from build123d import *

# Parameters (mm, degrees)
PAD_DEPTH       = 5
POCKET_DEPTH    = 5
POCKET001_DEPTH = 2.7
SKETCH001_R     = 6
PAD001_DEPTH    = 10
SKETCH003_R     = 1.75
POCKET002_DEPTH = 15.001
SKETCH_R        = 5.5
POCKET003_DEPTH = 0.28
SKETCH008_R     = 3.108339
PAD002_DEPTH    = 0.28


with BuildPart() as part:
    # Sketch002 → Pad (new body)
    with BuildSketch(Plane(origin=(0, 0, 0), x_dir=(1, 0, 0), z_dir=(0, 0, -1))):
        with BuildLine():
            ThreePointArc((-6.818582, 13.360649), (-8.459114, 12.387227), (-9.962838, 11.213468))
            ThreePointArc((-9.962838, 11.213468), (-11.40037, 11.226378), (-11.365355, 9.789214))
            ThreePointArc((-11.365355, 9.789214), (-12.514173, 8.270155), (-13.461245, 6.617771))
            ThreePointArc((-13.461245, 6.617771), (-14.797088, 6.086557), (-14.221642, 4.769163))
            ThreePointArc((-14.221642, 4.769163), (-14.712665, 2.9219), (-14.964788, 1.027192))
            ThreePointArc((-14.964788, 1.027192), (-15.999972, 0.029665), (-14.968494, -0.971693))
            ThreePointArc((-14.968494, -0.971693), (-14.718057, -2.894616), (-14.221642, -4.769163))
            ThreePointArc((-14.221642, -4.769163), (-14.797088, -6.086557), (-13.461245, -6.617771))
            ThreePointArc((-13.461245, -6.617771), (-12.514173, -8.270155), (-11.365355, -9.789214))
            ThreePointArc((-11.365355, -9.789214), (-11.40037, -11.226378), (-9.962838, -11.213468))
            ThreePointArc((-9.962838, -11.213468), (-8.459114, -12.387227), (-6.818582, -13.360649))
            ThreePointArc((-6.818582, -13.360649), (-6.307429, -14.704296), (-4.981567, -14.148639))
            ThreePointArc((-4.981567, -14.148639), (-3.026004, -14.691606), (-1.015045, -14.965617))
            ThreePointArc((-1.015045, -14.965617), (-0.016678, -15.999991), (0.983842, -14.9677))
            ThreePointArc((0.983842, -14.9677), (3.010688, -14.694753), (4.981567, -14.148639))
            ThreePointArc((4.981567, -14.148639), (6.307429, -14.704296), (6.818582, -13.360649))
            ThreePointArc((6.818582, -13.360649), (8.459114, -12.387227), (9.962838, -11.213468))
            ThreePointArc((9.962838, -11.213468), (11.40037, -11.226378), (11.365355, -9.789214))
            ThreePointArc((11.365355, -9.789214), (12.514173, -8.270155), (13.461245, -6.617771))
            ThreePointArc((13.461245, -6.617771), (14.797088, -6.086557), (14.221642, -4.769163))
            ThreePointArc((14.221642, -4.769163), (14.718057, -2.894616), (14.968494, -0.971693))
            ThreePointArc((14.968494, -0.971693), (15.999972, 0.029665), (14.964788, 1.027192))
            ThreePointArc((14.964788, 1.027192), (14.712665, 2.9219), (14.221642, 4.769163))
            ThreePointArc((14.221642, 4.769163), (14.797088, 6.086557), (13.461245, 6.617771))
            ThreePointArc((13.461245, 6.617771), (12.514173, 8.270155), (11.365355, 9.789214))
            ThreePointArc((11.365355, 9.789214), (11.40037, 11.226378), (9.962838, 11.213468))
            ThreePointArc((9.962838, 11.213468), (8.459114, 12.387227), (6.818582, 13.360649))
            ThreePointArc((6.818582, 13.360649), (6.307429, 14.704296), (4.981567, 14.148639))
            ThreePointArc((4.981567, 14.148639), (3.010688, 14.694753), (0.983842, 14.9677))
            ThreePointArc((0.983842, 14.9677), (-0.016678, 15.999991), (-1.015045, 14.965617))
            ThreePointArc((-1.015045, 14.965617), (-3.026004, 14.691606), (-4.981567, 14.148639))
            ThreePointArc((-4.981567, 14.148639), (-6.307429, 14.704296), (-6.818582, 13.360649))
        make_face()
    extrude(amount=PAD_DEPTH)

    # Sketch006 → Pocket (cut)
    with BuildSketch(Plane.XY):
        with BuildLine():
            ThreePointArc((-9.143797, 7.729592), (-11.061719, 4.581917), (-11.931287, 1))
            Line((-5.91608, 1), (-11.931287, 1))
            ThreePointArc((-4.890405, 3.476196), (-5.543277, 2.296102), (-5.91608, 1))
            Line((-9.143797, 7.729592), (-4.890405, 3.476196))
        make_face()
        with BuildLine():
            ThreePointArc((-11.931287, -1), (-11.061721, -4.581914), (-9.143802, -7.729585))
            Line((-4.890408, -3.476192), (-9.143802, -7.729585))
            ThreePointArc((-5.91608, -1), (-5.543277, -2.2961), (-4.890408, -3.476192))
            Line((-5.91608, -1), (-11.931287, -1))
        make_face()
        with BuildLine():
            ThreePointArc((-1, 11.931287), (-4.581912, 11.061722), (-7.729583, 9.143804))
            Line((-7.729583, 9.143804), (-3.476191, 4.890408))
            ThreePointArc((-1, 5.91608), (-2.296099, 5.543278), (-3.476191, 4.890408))
            Line((-1, 11.931287), (-1, 5.91608))
        make_face()
        with BuildLine():
            ThreePointArc((7.729588, 9.143799), (4.581915, 11.06172), (1, 11.931287))
            Line((1, 11.931287), (1, 5.91608))
            ThreePointArc((3.476194, 4.890406), (2.296101, 5.543277), (1, 5.91608))
            Line((7.729588, 9.143799), (3.476194, 4.890406))
        make_face()
        with BuildLine():
            ThreePointArc((9.143797, -7.729592), (11.061719, -4.581917), (11.931287, -1))
            Line((11.931287, -1), (5.91608, -1))
            ThreePointArc((4.890405, -3.476196), (5.543277, -2.296102), (5.91608, -1))
            Line((4.890405, -3.476196), (9.143797, -7.729592))
        make_face()
        with BuildLine():
            ThreePointArc((1, -11.931287), (4.581912, -11.061722), (7.729583, -9.143804))
            Line((3.476191, -4.890408), (7.729583, -9.143804))
            ThreePointArc((1, -5.91608), (2.296099, -5.543278), (3.476191, -4.890408))
            Line((1, -5.91608), (1, -11.931287))
        make_face()
        with BuildLine():
            ThreePointArc((-7.729589, -9.143799), (-4.581916, -11.06172), (-1, -11.931287))
            Line((-1, -5.91608), (-1, -11.931287))
            ThreePointArc((-3.476194, -4.890406), (-2.296101, -5.543277), (-1, -5.91608))
            Line((-3.476194, -4.890406), (-7.729589, -9.143799))
        make_face()
        with BuildLine():
            ThreePointArc((11.931287, 1), (11.061721, 4.581914), (9.143802, 7.729586))
            Line((9.143802, 7.729586), (4.890407, 3.476193))
            ThreePointArc((5.91608, 1), (5.543277, 2.2961), (4.890407, 3.476193))
            Line((11.931287, 1), (5.91608, 1))
        make_face()
    extrude(amount=-POCKET_DEPTH, mode=Mode.SUBTRACT)

    # Sketch007 (on Face34 of Pad) → Pocket001 (cut)
    with BuildSketch(Plane(origin=(0, 0, -5), x_dir=(1, 0, 0), z_dir=(0, 0, -1))):
        Polygon((3.3, -1.918967), (3.311874, 1.8984), (0.011874, 3.817367), (-3.3, 1.918967), (-3.311874, -1.8984), (-0.011874, -3.817367), align=None)
    extrude(amount=-POCKET001_DEPTH, mode=Mode.SUBTRACT)

    # Sketch001 (on Face33 of Pad) → Pad001 (join)
    with BuildSketch(Plane.XY):
        Circle(SKETCH001_R)
    extrude(amount=PAD001_DEPTH)

    # Sketch003 (on Face74 of Pad001) → Pocket002 (cut, through all)
    with BuildSketch(Plane.XY.offset(10)):
        Circle(SKETCH003_R)
    extrude(amount=-POCKET002_DEPTH, mode=Mode.SUBTRACT)

    # Sketch (on Face74 of Pocket002) → Pocket003 (cut)
    with BuildSketch(Plane.XY.offset(10)):
        Circle(SKETCH_R)
    extrude(amount=-POCKET003_DEPTH, mode=Mode.SUBTRACT)

    # Sketch008 (on Face4 of Pocket003) → Pad002 (join)
    with BuildSketch(Plane.XY.offset(-2.3)):
        Circle(SKETCH008_R)
    extrude(amount=PAD002_DEPTH)


solid = part.part
Check sheet for the modelled part. Datum: model origin and axes. Units: mm. A direction names the side the tool comes from. Round coordinates to 2 decimals unless told otherwise and drop trailing zeros. Order: outer loops, then holes, each group sorted by start corner. A loop starts at its lowest first (then second) coordinate and runs counter-clockwise, first axis right, second up.
(1) Scan lines: probe 1 along Y at (x, z) = (0, 9.9); probe 2 along X at (y, z) = (10, -2.25); probe 3 along Y at (x, z) = (-8.5, -3.5). Record each from-to range of solid material in increasing order.
(2) Cross-section at B-B, the plane z = 2.25. Enter the section's corners in (x, y), and give its area (3 significant figures).
(3) Cross-section at C-C, the plane y = 0. Enter the section's corners in (x, z), and give its area (3 significant figures).
(4) Cross-section at A-A, the plane x = 0.5. Enter the section's corners in (y, z), and give its area (3 significant figures).
(5) Cross-section at D-D, the plane z = -3.5. State how many separate pieces and enclosed holes the cut face has, and give its area (3 significant figures).
(6) Go/stop test with flat-tipped pins: P1, Ø5.5, axis at x = -8.5, z = -2, coming from the -Y side; P2, Ø2, axis at y = 2.5, z = -2, coming from the -X side; P3, Ø5, axis at x = 4.5, z = 7, coming from the -Y side; P4, Ø2, axis at x = 2.5, y = 10, coming from the -Z side. Record where each tip stops, or that it passes through.
(7) Draft check along Y on faces 6 (the cylindrical face through (-16, 0, -2)), 7 (the flat face through (9, 1, -2)), 8 (the flat face through (-4, 0, -5)). Enter one of: pulls with the +Y half, pulls with the -Y half, needs draft (parallel to the pull), parting line crosses it, or undercut.
(8) Access from +Z, -Z, +X, -X, +Y, -Y to the whole of each face (thin tool, end or side, straight path). Record for faces 1 (the cylindrical face through (2.98, 14.7, -2.46)), 2 (the flat face through (5.573, -6.987, -2.465)), 3 (the cylindrical face through (1.617, -0.67, 3.932)), 4 (the cylindrical face through (-2.998, -14.697, -2.465)), 5 (the cylindrical face through (-14.707, -2.948, -2.465)).
Check sheet entries:
1. probe 1: y = -6 to -5.5, 5.5 to 6
1. probe 2: x = -11.54 to -6.58, -1 to 1, 6.58 to 11.54
1. probe 3: y = -12.36 to -7.09, -1 to 1, 7.09 to 12.36
2. outline: circle Ø12 at (0, 0); hole circle Ø3.5 at (0, 0)
2. area: 103 mm2
3. outline: (-16, -5) - (-3.31, -5) - (-3.31, -2.3) - (3.31, -2.3) - (3.31, -5) - (16, -5) - (16, 0) - (6, 0) - (6, 10) - (5.5, 10) - (5.5, 9.72) - (1.75, 9.72) - (1.75, -2.02) - (-1.75, -2.02) - (-1.75, 9.72) - (-5.5, 9.72) - (-5.5, 10) - (-6, 10) - (-6, 0) - (-16, 0) - close
3. area: 218 mm2
4. outline: (-15.86, -5) - (-3.53, -5) - (-3.53, -2.3) - (3.52, -2.3) - (3.52, -5) - (15.86, -5) - (15.86, 0) - (5.98, 0) - (5.98, 10) - (5.48, 10) - (5.48, 9.72) - (1.68, 9.72) - (1.68, -2.02) - (-1.68, -2.02) - (-1.68, 9.72) - (-5.48, 9.72) - (-5.48, 10) - (-5.98, 10) - (-5.98, 0) - (-15.86, 0) - close
4. area: 217 mm2
5. separate pieces: 1
5. enclosed holes: 9
5. area: 453 mm2
6. P1: stops at y = -14.79
6. P2: stops at x = -14.92
6. P3: stops at y = -5.66
6. P4: passes through
7. face 6: parting line crosses it
7. face 7: undercut
7. face 8: needs draft
8. face 1: +Z, -Z, +Y
8. face 2: +Z, -Z
8. face 3: +Z
8. face 4: +Z, -Z, -Y
8. face 5: +Z, -Z, -X
